Check sheet for the modelled part. Datum: model origin and axes. Units: mm. Face numbers are marked on the shaded views. A direction names the side the tool comes from. Round coordinates to 2 decimals unless told otherwise and drop trailing zeros. Order: outer loops, then holes, each group sorted by start corner. A loop starts at its lowest first (then second) coordinate and runs counter-clockwise, first axis right, second up.
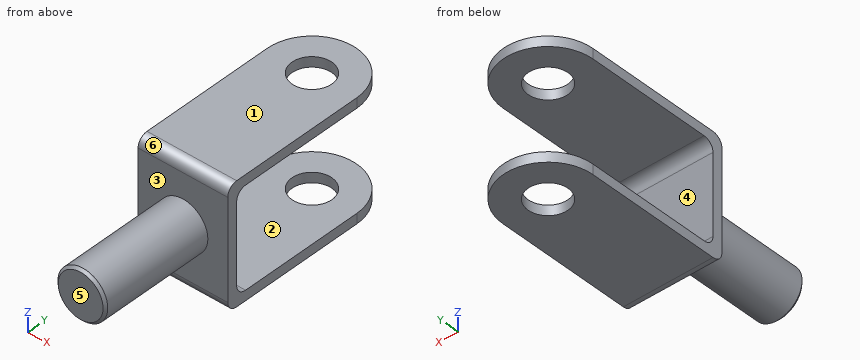
Autodesk Inventor part; units mm, degrees
ref_plane "YZ Plane" through (0, 0, 0) normal (1, 0, 0) x (0, 1, 0)
ref_plane "XZ Plane" through (0, 0, 0) normal (0, 1, 0) x (-1, 0, 0)
ref_plane "XY Plane" through (0, 0, 0) normal (0, 0, 1) x (1, 0, 0)
sketch "Sketch1" plane through (0, 0, 0) normal (0, 1, 0) x (-1, 0, 0)
  line L0 (9, 12) -> (-9, 12)
  line L1 (-9, 12) -> (-9, -12)
  line L2 (-9, -12) -> (9, -12)
  line L3 (9, -12) -> (9, 12)
  line L4 (9, 12) -> (-9, -12) construction
  line L5 (-9, 12) -> (9, -12) construction
  point P0 (0, 0)
  dimension "d0" = 24
  dimension "d1" = 18
extrude "Extrusion1" add sketch "Sketch1" along normal blind 2
sketch "Sketch2" plane through (0, 2, 0) normal (0, 1, 0) x (1, 0, 0)
  line L0 (-9, 12) -> (-9, -12)
  line L1 (9, -12) -> (9, 12)
  line L2 (-9, -12) -> (9, -12)
  line L3 (9, -12) -> (9, -10)
  line L4 (9, -10) -> (-9, -10)
  line L5 (-9, -10) -> (-9, -12)
  line L6 (9, 12) -> (-9, 12)
  line L7 (-9, 12) -> (9, 12)
  line L8 (9, 12) -> (9, 10)
  line L9 (9, 10) -> (-9, 10)
  line L10 (-9, 10) -> (-9, 12)
  point P0 (0, 0)
  dimension "d4" = 2
  dimension "d5" = 2
extrude "Extrusion2" add sketch "Sketch2" along normal blind 36 contours L6 L1 L9 L0 | L4 L1 L2 L0
sketch "Sketch5" plane through (-9, 0, 12) normal (0, 0, 1) x (1, 0, 0)
  line L0 (0, 29) -> (18, 29)
  line L1 (0, 38) -> (18, 38)
  arc A0 (18, 29) -> (0, 29) centre (9, 29) ccw
  circle A1 centre (9, 29) radius 4
  line L2 (0, 0) -> (0, 38)
  line L3 (0, 29) -> (0, 38)
  line L4 (18, 38) -> (0, 38)
  line L5 (0, 38) -> (18, 38)
  line L6 (18, 38) -> (18, 29)
  point P0 (9, 0)
  dimension "d16" = 9
  dimension "d17" = 8
extrude "Extrusion4" cut sketch "Sketch5" against normal blind 40 contours A1 L0 | L0 A1 | A0 L1 L6 | A0 L2 L1
sketch "Sketch6" plane through (0, 0, 0) normal (0, -1, 0) x (1, 0, 0)
  circle A0 centre (0, 0) radius 4
  dimension "d20" = 8
extrude "Extrusion5" cut sketch "Sketch6" against normal blind 40
fillet "Fillet1" radius 2 4 edges at (0, 0, 12) (0, 0, -12) (0, 2, 10) (0, 2, -10)
sketch "Sketch11" plane through (0, 2, 0) normal (0, 1, 0) x (1, 0, 0)
  circle A0 centre (0, 0) radius 5
  dimension "d29" = 10
extrude "Extrusion7" add sketch "Sketch11" against normal blind 25
thread "Thread2"
chamfer "Chamfer1" distance 0.5 angle 45 1 edges at (-5, -23, 0)
properties part number "Giá đỡ ròng rọc"
Item 1: Sectioned sample at C-C (x = -3.25). State how many separate pieces and enclosed holes the cut face has, and give its area (3 significant figures).
Answer:
separate pieces: 3
enclosed holes: 0
area: 345 mm2
Item 2: Access from +Z, -Z, +X, -X, +Y, -Y to the whole of each face (thin tool, end or side, straight path). Record for the marked faces 1, 2 and 3.
Answer:
face 1: +Z, +X, -X, +Y, -Y
face 2: +X, -X, +Y
face 3: -Y
Item 3: Sectioned sample at B-B (y = 6). Record the cut outline in (x, z).
Answer:
outline: (-9, -12) - (9, -12) - (9, -10) - (-9, -10) - close; (-9, 10) - (9, 10) - (9, 12) - (-9, 12) - close
Item 4: Release check for a two-part mould opening along Z. For the marked faces 4, 5 and 6 record: released by +Z, released by -Z, zero draft, split by the parting line, or undercut.
Answer:
face 4: undercut
face 5: zero draft
face 6: released by +Z
Item 5: Sectioned sample at A-A (x = 0). Record the cut outline in (y, z), and give its area (3 significant figures).
Answer:
outline: (-23, -4.5) - (-22.5, -5) - (0, -5) - (0, -10) arc R2 ccw to (2, -12) - (25, -12) - (25, -10) - (4, -10) arc R2 cw to (2, -8) - (2, 8) arc R2 cw to (4, 10) - (25, 10) - (25, 12) - (2, 12) arc R2 ccw to (0, 10) - (0, 5) - (-22.5, 5) - (-23, 4.5) - close; (33, -12) - (38, -12) - (38, -10) - (33, -10) - close; (33, 10) - (38, 10) - (38, 12) - (33, 12) - close
area: 390 mm2
Item 6: Go/stop test with flat-tipped pins: P1, Ø6, axis at x = -2, z = -4.5, coming from the -Y side; P2, Ø12, axis at y = 19.5, z = -1.5, coming from the +X side; P3, Ø4, axis at x = -4.5, z = -1.5, coming from the +Y side; P4, Ø4, axis at y = -16.5, z = 1, coming from the -X side. Record where each tip stops, or that it passes through.
Answer:
P1: stops at y = -23
P2: passes through
P3: stops at y = 2
P4: stops at x = -5
Item 7: Scan lines: line 1 along Z through (x, y) = (-8, 17); line 2 along X through (y, z) = (29, 11.6); line 3 along Y through (x, z) = (0, -2.25). Record each from-to range of solid material in increasing order.
Answer:
line 1: z = -12 to -10, 10 to 12
line 2: x = -9 to -4, 4 to 9
line 3: y = -23 to 2
